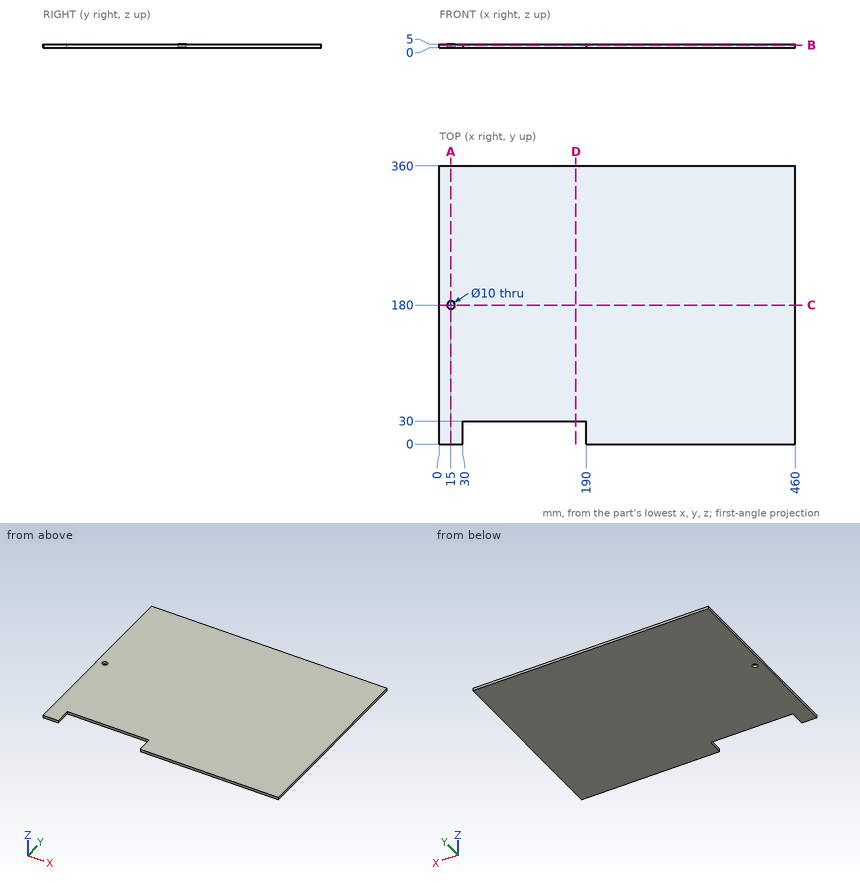
Geometry: see drawing. Coordinates: mm, zero at the bounding-box minimum. Round coordinates to 2 decimals unless told otherwise and drop trailing zeros. Loops run counter-clockwise (first coordinate to the right, second up) from the corner with the lowest first, then second, coordinate; pieces in that order, holes last. Notation, with made-up numbers: (-39, -33.75) - (20, -33.75) arc R24 cw to (20, -23.75) - close; hole circle Ø11 at (79, 32.5). An arc over 180 degrees is marked (long way). Write item = value, one per line. Start each with the question number.
(1) Section query C-C, the plane y = 180. Output: boundary loops of the cut face in (x, z).
(2) Section query D-D, the plane x = 176.5. Output: boundary loops of the cut face in (y, z).
(3) Ray query, line 1 along Y through (x, z) = (15, 2.7); line 2 along Y through (x, z) = (124.5, 0.5). Return the intervals inside material, ascending. Write a range as from..to.
(4) Section query B-B, the plane z = 3.45. Output: boundary loops of the cut face in (x, y).
(5) Section query A-A, the plane x = 15. Output: boundary loops of the cut face in (y, z), plus the area to 3 significant figures.
Conclusion:
q1.outline = (0, 0) - (10, 0) - (10, 5) - (0, 5) - close; (20, 0) - (460, 0) - (460, 5) - (20, 5) - close
q2.outline = (30, 0) - (360, 0) - (360, 5) - (30, 5) - close
q3.line_1 = 0..175, 185..360
q3.line_2 = 30..360
q4.outline = (0, 0) - (30, 0) - (30, 30) - (190, 30) - (190, 0) - (460, 0) - (460, 360) - (0, 360) - close; hole circle Ø10 at (15, 180)
q5.outline = (0, 0) - (175, 0) - (175, 5) - (0, 5) - close; (185, 0) - (360, 0) - (360, 5) - (185, 5) - close
q5.area = 1,750 mm2
